from build123d import *

# Parameters (mm, degrees)
SKETCH_1_R        = 1.6
SKETCH_1_R_2      = 1.1
SKETCH_1_W        = 2.5
SKETCH_1_H        = 12
SKETCH_1_W_2      = 18
SKETCH_1_H_2      = 18
EXTRUDE_284_DEPTH = 1.5
SKETCH_2_R        = 1.1
D2P2_DEPTH        = 1.5


with BuildPart() as part:
    # 草图1 → Extrude 284 (new body)
    with BuildSketch(Plane.XY):
        Polygon((-22, 4), (22, 4), (28, 10), (28, 60), (22, 66), (-22, 66), (-28, 60), (-28, 10), align=None)
        with Locations((-12, 8)):
            Circle(SKETCH_1_R, mode=Mode.SUBTRACT)
        with Locations((-24, 62)):
            Circle(SKETCH_1_R_2, mode=Mode.SUBTRACT)
        with Locations((12, 8)):
            Circle(SKETCH_1_R, mode=Mode.SUBTRACT)
        with Locations((24, 62)):
            Circle(SKETCH_1_R_2, mode=Mode.SUBTRACT)
        with Locations((-14, 24)):
            Circle(SKETCH_1_R_2, mode=Mode.SUBTRACT)
        with Locations((-14, 52)):
            Circle(SKETCH_1_R_2, mode=Mode.SUBTRACT)
        with Locations((14, 24)):
            Circle(SKETCH_1_R_2, mode=Mode.SUBTRACT)
        with Locations((14, 52)):
            Circle(SKETCH_1_R_2, mode=Mode.SUBTRACT)
        with Locations((-17, 21)):
            Circle(SKETCH_1_R_2, mode=Mode.SUBTRACT)
        with Locations((-17, 55)):
            Circle(SKETCH_1_R_2, mode=Mode.SUBTRACT)
        with Locations((17, 21)):
            Circle(SKETCH_1_R_2, mode=Mode.SUBTRACT)
        with Locations((17, 55)):
            Circle(SKETCH_1_R_2, mode=Mode.SUBTRACT)
        with Locations((-24, 38)):
            Rectangle(SKETCH_1_W, SKETCH_1_H, mode=Mode.SUBTRACT)
        with Locations((24, 38)):
            Rectangle(SKETCH_1_W, SKETCH_1_H, mode=Mode.SUBTRACT)
        with Locations((0, 38)):
            Rectangle(SKETCH_1_W_2, SKETCH_1_H_2, mode=Mode.SUBTRACT)
        Polygon((-9, 16), (9, 16), (0, 23), align=None, mode=Mode.SUBTRACT)
    extrude(amount=EXTRUDE_284_DEPTH)

    # 草图2 → 外拉钢索两孔_D2p2 (cut)
    with BuildSketch(Plane.XY):
        with Locations((-14, 62)):
            Circle(SKETCH_2_R)
        with Locations((14, 62)):
            Circle(SKETCH_2_R)
    extrude(amount=D2P2_DEPTH, mode=Mode.SUBTRACT)


solid = part.part
Design review of the part built by this model. Coordinates are the model's own, in mm. A direction names the side the tool comes from. Give positions to 0.01 mm unless a question says otherwise; leave off trailing zeros. Loops run counter-clockwise (first coordinate to the right, second up) from the corner with the lowest first, then second, coordinate; pieces in that order, holes last. Notation, with made-up numbers: M 50.25,84.25 L 102.25,84.25 A17 ccw 102.25,94.25 Z; hole C 6.5,72.5 d8. An arc over 180 degrees is marked long. One line per question, with ' | ' between items. Start each with the question number.
1. Add section B-B (x = -24). Write out the cut boundary in (y, z).
2. Add section A-A (y = 34). Write out the cut boundary in (x, z).
3. The part is to be moulded in two halves that separate along X. For faces 3 (the face through (-25.25, 38, 1)), 4 (the face through (-17.14, 56.09, 0.74)), 5 (the face through (-28, 35, 1)), 6 (the face through (28, 35, 1)), say which applies: released by +X, released by -X, zero draft, split by the parting line, or undercut.
4. To check wall thickness, follow L1, parallel to Y at x = 14, z = 0.3; L2, parallel to X at y = 42, z = 0.7; L3, parallel to Y at x = -17, z = 0.7. State the ranges of each line that lie inside material, in increasing order.
5. For faces 1 (the face through (0, 47, 1)), 2 (the face through (-25, 7, 1)), list the 3-axis set-ups (+Z, -Z, +X, -X, +Y, -Y) from which the entire face can be reached by the end or side of a thin tool; tool diameter is ignored.
6. Add section C-C (y = 62). Write out the cut boundary in (x, z), plus the area to 3 significant figures.
7. Add section D-D (y = 52). Write out the cut boundary in (x, z).
8. Insertion check: P1, Ø1.3, axis at x = 14, y = 62, coming from the -Z side. The pin has a flat end and moves straight along its axis. Give the tip position at first contact, or say it passes through.
Worked out:
1) outline: M 6,0 L 32,0 L 32,1.5 L 6,1.5 Z; M 44,0 L 60.9,0 L 60.9,1.5 L 44,1.5 Z; M 63.1,0 L 64,0 L 64,1.5 L 63.1,1.5 Z
2) outline: M -28,0 L -25.25,0 L -25.25,1.5 L -28,1.5 Z; M -22.75,0 L -9,0 L -9,1.5 L -22.75,1.5 Z; M 9,0 L 22.75,0 L 22.75,1.5 L 9,1.5 Z; M 25.25,0 L 28,0 L 28,1.5 L 25.25,1.5 Z
3) face 3: undercut | face 4: undercut | face 5: released by -X | face 6: released by +X
4) L1: y = 4 to 22.9, 25.1 to 50.9, 53.1 to 60.9, 63.1 to 66 | L2: x = -28 to -25.25, -22.75 to -9, 9 to 22.75, 25.25 to 28 | L3: y = 4 to 19.9, 22.1 to 53.9, 56.1 to 66
5) face 1: +Z, -Z | face 2: +Z, -Z, -X, -Y
6) outline: M -26,0 L -25.1,0 L -25.1,1.5 L -26,1.5 Z; M -22.9,0 L -15.1,0 L -15.1,1.5 L -22.9,1.5 Z; M -12.9,0 L 12.9,0 L 12.9,1.5 L -12.9,1.5 Z; M 15.1,0 L 22.9,0 L 22.9,1.5 L 15.1,1.5 Z; M 25.1,0 L 26,0 L 26,1.5 L 25.1,1.5 Z | area: 64.8 mm²
7) outline: M -28,0 L -15.1,0 L -15.1,1.5 L -28,1.5 Z; M -12.9,0 L 12.9,0 L 12.9,1.5 L -12.9,1.5 Z; M 15.1,0 L 28,0 L 28,1.5 L 15.1,1.5 Z
8) P1: passes through
